```python
from build123d import *

# Parameters (mm, degrees)
SKETCH_1_W      = 26.4
SKETCH_1_H      = 45.5
EXTRUDE_1_DEPTH = 16.5
FILLET_1_R      = 3
SKETCH_2_R      = 3
SKETCH_2_R_2    = 1.5
SKETCH_2_R_3    = 4.5
EXTRUDE_2_DEPTH = 3.6
FILLET_2_R      = 1


with BuildPart() as part:
    # 草圖1 → 填料-伸長1 (new body)
    with BuildSketch(Plane.XY):
        with Locations((13.2, 22.75)):
            Rectangle(SKETCH_1_W, SKETCH_1_H)
    extrude(amount=EXTRUDE_1_DEPTH)

    # 圓角1
    fillet_1_edges = [part.edges().sort_by_distance(p)[0] for p in [
        (26.4, 22.75, 16.5),
        (0, 22.75, 16.5),
        (26.4, 22.75, 0),
        (0, 22.75, 0),
    ]]
    fillet(fillet_1_edges, radius=FILLET_1_R)

    # 草圖2 → 填料-伸長2 (add)
    with BuildSketch(Plane(origin=(0, 45.5, 0), x_dir=(1, 0, 0), z_dir=(0, 1, 0))):
        with Locations((7.4, -8.25)):
            Circle(SKETCH_2_R)
        with Locations((7.4, -8.25)):
            Circle(SKETCH_2_R_2, mode=Mode.SUBTRACT)
        with Locations((19.4, -8.25)):
            Circle(SKETCH_2_R_3)
        with Locations((19.4, -8.25)):
            Circle(SKETCH_2_R, mode=Mode.SUBTRACT)
    extrude(amount=EXTRUDE_2_DEPTH)

    # 圓角2
    fillet_2_edges = [part.edges().sort_by_distance(p)[0] for p in [
        (0, 0, 8.25),
        (0, 45.5, 8.25),
        (13.2, 0, 0),
        (26.4, 0, 8.25),
        (13.2, 0, 16.5),
        (25.521320344, 0, 15.621320344),
        (25.521320344, 0, 0.878679656),
        (0.878679656, 0, 15.621320344),
        (0.878679656, 0, 0.878679656),
        (13.2, 45.5, 0),
        (13.2, 45.5, 16.5),
        (26.4, 45.5, 8.25),
        (25.521320344, 45.5, 15.621320344),
        (25.521320344, 45.5, 0.878679656),
        (0.878679656, 45.5, 15.621320344),
        (0.878679656, 45.5, 0.878679656),
    ]]
    fillet(fillet_2_edges, radius=FILLET_2_R)


solid = part.part
```
Check sheet for the modelled part. Datum: model origin and axes. Units: mm. A direction names the side the tool comes from. Round coordinates to 2 decimals unless told otherwise and drop trailing zeros. Order: outer loops, then holes, each group sorted by start corner. A loop starts at its lowest first (then second) coordinate and runs counter-clockwise, first axis right, second up. Notation, with made-up numbers: (44, 67.25) - (50, 67.25) arc R10 ccw to (50, 84.25) - close; hole circle Ø10 at (80, 69.5). An arc over 180 degrees is marked (long way). Write item = value, one per line.
Q1. Section check A-A (x = 19.4). Record the boundary of the cut face in (y, z), and give its area (3 significant figures).
Computed:
outline = (0, 1) arc R1 ccw to (1, 0) - (44.5, 0) arc R1 ccw to (45.5, 1) - (45.5, 3.75) - (49.1, 3.75) - (49.1, 5.25) - (45.5, 5.25) - (45.5, 11.25) - (49.1, 11.25) - (49.1, 12.75) - (45.5, 12.75) - (45.5, 15.5) arc R1 ccw to (44.5, 16.5) - (1, 16.5) arc R1 ccw to (0, 15.5) - close
area = 761 mm^2
Q2. Draft check along Z on faces 3 (the face through (25.54, 23.05, 0.9)), 4 (the face through (0, 22, 8)), 5 (the face through (21.01, 47.27, 5.72)). Enter one of: pulls with the +Z half, pulls with the -Z half, needs draft (parallel to the pull), parting line crosses it, or undercut.
Computed:
face_3 = pulls with the -Z half
face_4 = needs draft
face_5 = undercut
Q3. Section check D-D (x = 11). Record the boundary of the cut face in (y, z).
Computed:
outline = (0, 1) arc R1 ccw to (1, 0) - (44.5, 0) arc R1 ccw to (45.5, 1) - (45.5, 15.5) arc R1 ccw to (44.5, 16.5) - (1, 16.5) arc R1 ccw to (0, 15.5) - close
Q4. Go/stop test with a flat-tipped pin: pin 1 (1.8 mm diameter, centred on x = 20.5, z = 7, fed in from +Y). Record where the tip stops, or that it passes through.
Computed:
pin_1 = 45.5
Q5. Tool access check on faces 1 (the face through (5.19, 47.27, 6.22)), 2 (the face through (26.4, 22, 8)). Record the directions out of +Z, -Z, +X, -X, +Y, -Y that give a thin tool (end or side, any length) a straight path to the whole face; none if there is none.
Computed:
face_1 = +Y
face_2 = +Z, -Z, +X, +Y, -Y
Q6. Thickness scan on line 1 along X through (y, z) = (46.75, 8.25); line 2 along Z through (x, y) = (19.4, 46.8); line 3 along Y through (x, z) = (2.25, 6.75). Record the ranges inside material, lowest first.
Computed:
line_1 = 4.4 to 5.9, 8.9 to 10.4, 14.9 to 16.4, 22.4 to 23.9
line_2 = 3.75 to 5.25, 11.25 to 12.75
line_3 = 0 to 45.5
Q7. Section check B-B (z = 8.25). Record the boundary of the cut face in (x, y), and give its area (3 significant figures).
Computed:
outline = (0, 1) arc R1 ccw to (1, 0) - (25.4, 0) arc R1 ccw to (26.4, 1) - (26.4, 44.5) arc R1 ccw to (25.4, 45.5) - (23.9, 45.5) - (23.9, 49.1) - (22.4, 49.1) - (22.4, 45.5) - (16.4, 45.5) - (16.4, 49.1) - (14.9, 49.1) - (14.9, 45.5) - (10.4, 45.5) - (10.4, 49.1) - (8.9, 49.1) - (8.9, 45.5) - (5.9, 45.5) - (5.9, 49.1) - (4.4, 49.1) - (4.4, 45.5) - (1, 45.5) arc R1 ccw to (0, 44.5) - close
area = 1,220 mm^2
Q8. Section check C-C (y = 18.5). Record the boundary of the cut face in (x, z), and give its area (3 significant figures).
Computed:
outline = (0, 3) arc R3 ccw to (3, 0) - (23.4, 0) arc R3 ccw to (26.4, 3) - (26.4, 13.5) arc R3 ccw to (23.4, 16.5) - (3, 16.5) arc R3 ccw to (0, 13.5) - close
area = 428 mm^2
